```python
from build123d import *

# Parameters (mm, degrees)
F0_W     = 132.6081287116
F0_H     = 90.7132923603
F1_DEPTH = 76.2
F3_W     = 279.7318845987
F3_H     = 160.2330692112
F4_DEPTH = 76.2
F5_T     = -2.54


with BuildPart() as f1:
    # F0 (on Right) → F1 (new body)
    with BuildSketch(Plane.YZ):
        with Locations((-39.4802326337, -12.3488530517)):
            Rectangle(F0_W, F0_H)
    extrude(amount=F1_DEPTH)


with BuildPart() as f4:
    # F3 (on Top) → F4 (new body)
    with BuildSketch(Plane.XY):
        with Locations((-21.0741087794, 28.8107972592)):
            Rectangle(F3_W, F3_H)
    extrude(amount=F4_DEPTH)

    # F5
    f5_openings = [f4.faces().sort_by_distance(p)[0] for p in [
        (-21.074109, 28.810797, 76.2),
    ]]
    offset(amount=F5_T, openings=f5_openings)


solid = f4.part
```
Verification items for the finished model (mm, model axes). A direction names the side the tool comes from. Give positions to 0.01 mm unless a question says otherwise; leave off trailing zeros. Order: outer loops, then holes, each group sorted by start corner. A loop starts at its lowest first (then second) coordinate and runs counter-clockwise, first axis right, second up. Notation, with made-up numbers: (-4.5, -21.5) -> (1.5, -21.5) arc R27 cw to (1.5, 2.5) -> close; hole circle Ø3 at (24, 17.25). An arc over 180 degrees is marked (long way). Use a Markdown table: item, result.
1) Mould release check, pull along X, two halves, no side actions. Record for faces 1 (the flat face through (116.252, 28, 39)), 2 (the flat face through (-23, 108.927, 38)), 3 (the flat face through (-160.94, 28, 38)): pulls with the +X half, pulls with the -X half, needs draft (parallel to the pull), parting line crosses it, or undercut.
Results:
| item | result |
|---|---|
| face 1 | undercut |
| face 2 | needs draft |
| face 3 | pulls with the -X half |
2) Material ranges on probe 1 along Y at (x, z) = (33, 60.5); probe 2 along X at (y, z) = (55, 64); probe 3 along Z at (x, y) = (-125, -38), recorded low to high.
Results:
| item | result |
|---|---|
| probe 1 | -51.31 to -48.77, 106.39 to 108.93 |
| probe 2 | -160.94 to -158.4, 116.25 to 118.79 |
| probe 3 | 0 to 2.54 |
3) Section check A-A, the plane z = 24.5. Record the boundary of the cut face in (x, y), then the cut area to 3 significant figures.
Results:
| item | result |
|---|---|
| outline | (-160.94, -51.31) -> (118.79, -51.31) -> (118.79, 108.93) -> (-160.94, 108.93) -> close; hole (-158.4, -48.77) -> (116.25, -48.77) -> (116.25, 106.39) -> (-158.4, 106.39) -> close |
| area | 2,210 mm² |
4) Tool access check on faces 4 (the flat face through (-23, 30, 0)), 5 (the flat face through (-23, 30, 2.54)). Record the directions out of +Z, -Z, +X, -X, +Y, -Y that give a thin tool (end or side, any length) a straight path to the whole face; none if there is none.
Results:
| item | result |
|---|---|
| face 4 | -Z, +X, -X, +Y, -Y |
| face 5 | +Z |
5) Section check B-B, the plane y = 66.5. Record the boundary of the cut face in (x, z).
Results:
| item | result |
|---|---|
| outline | (-160.94, 0) -> (118.79, 0) -> (118.79, 76.2) -> (116.25, 76.2) -> (116.25, 2.54) -> (-158.4, 2.54) -> (-158.4, 76.2) -> (-160.94, 76.2) -> close |
6) Depth check by flat-ended pin: pin 1 Ø3 at (x, y) = (85, -15.5) entering from +Z. Enter the tip coordinate at first touch or a pass-through.
Results:
| item | result |
|---|---|
| pin 1 | z = 2.54 |
7) Section check C-C, the plane x = -48. Record the boundary of the cut face in (y, z).
Results:
| item | result |
|---|---|
| outline | (-51.31, 0) -> (108.93, 0) -> (108.93, 76.2) -> (106.39, 76.2) -> (106.39, 2.54) -> (-48.77, 2.54) -> (-48.77, 76.2) -> (-51.31, 76.2) -> close |
